from build123d import *

# Parameters (mm, degrees)
IZIM1_R                     = 125
Y_KSEKLIK_EKSTR_ZYON2_DEPTH = 400
IZIM2_R                     = 530
KES_EKSTR_ZYON1_DEPTH       = 150
IZIM3_R                     = 540
Y_KSEKLIK_EKSTR_ZYON3_DEPTH = 300


with BuildPart() as part:
    # Çizim1 → Yükseklik-Ekstrüzyon2 (new body)
    with BuildSketch(Plane(origin=(0, 0, 0), x_dir=(1, 0, 0), z_dir=(0, 1, 0))):
        with BuildLine():
            Line((-900, 700), (-900, -700))
            ThreePointArc((-900, -700), (-841.421356237, -841.421356237), (-700, -900))
            Line((-700, -900), (700, -900))
            ThreePointArc((700, -900), (841.421356237, -841.421356237), (900, -700))
            Line((900, -700), (900, 700))
            ThreePointArc((900, 700), (841.421356237, 841.421356237), (700, 900))
            Line((700, 900), (-700, 900))
            ThreePointArc((-700, 900), (-841.421356237, 841.421356237), (-900, 700))
        make_face()
        with Locations((-550, 550)):
            Circle(IZIM1_R, mode=Mode.SUBTRACT)
        with Locations((550, 550)):
            Circle(IZIM1_R, mode=Mode.SUBTRACT)
        with Locations((-550, -550)):
            Circle(IZIM1_R, mode=Mode.SUBTRACT)
        with Locations((550, -550)):
            Circle(IZIM1_R, mode=Mode.SUBTRACT)
    extrude(amount=Y_KSEKLIK_EKSTR_ZYON2_DEPTH)

    # Çizim2 → Kes-Ekstrüzyon1 (cut)
    with BuildSketch(Plane.XZ):
        Circle(IZIM2_R)
    extrude(amount=-KES_EKSTR_ZYON1_DEPTH, mode=Mode.SUBTRACT)

    # Çizim3 → Yükseklik-Ekstrüzyon3 (add)
    with BuildSketch(Plane.XZ.offset(-150)):
        Circle(IZIM3_R)
    extrude(amount=Y_KSEKLIK_EKSTR_ZYON3_DEPTH)


solid = part.part
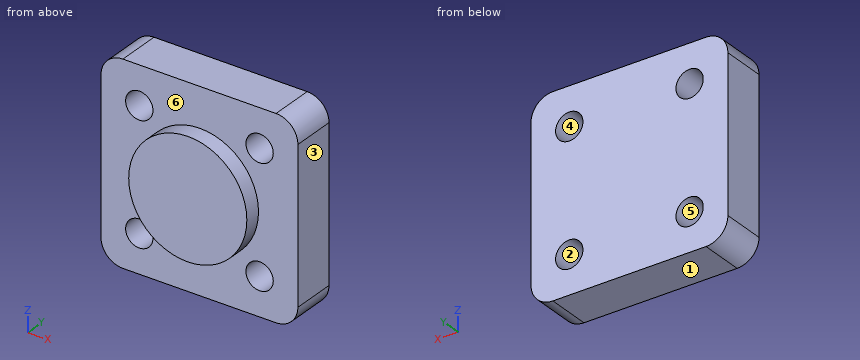
CAD build for the part. Positions are in the model's coordinates, mm. Face numbers are marked on the shaded views. A direction names the side the tool comes from. Coordinates: 2 decimals unless noted, no trailing zeros. Write each loop counter-clockwise with the first axis right and the second up, starting at its lowest first coordinate (ties: lowest second). Pieces come first, ordered by that corner, then holes. Notation, with made-up numbers: M 36.5,-29 L 45.5,-29 A7 ccw 45.5,-21 Z; hole C 71,50 d9. An arc over 180 degrees is marked long. Return JSON: item names as keys, results as strings.
Item 1: Slice it at C-C, the plane z = 288. Write the cut outline in (x, y).
Findings below:
{"outline": "M -900,0 L -456.79,0 L -456.79,-150 L 456.79,-150 L 456.79,0 L 900,0 L 900,400 L -900,400 Z"}
Item 2: Drop flat-ended pins along their axis: pin 1 Ø2 at (y, z) = (-77, -168) entering from -X; pin 2 Ø5 at (x, z) = (-351.5, -675) entering from -Y. Give the stop position or say it passes through.
Findings below:
{"pin 1": "stops at x = -513.53", "pin 2": "stops at y = 0"}
Item 3: Two-plate mould, pull along Z, no slides. Class the marked faces 1, 2, 3 and 4: +Z half, -Z half, draft (parallel to the pull), parting line (faces both ways), or undercut.
Findings below:
{"face 1": "-Z half", "face 2": "undercut", "face 3": "draft", "face 4": "undercut"}
Item 4: Probe line 1 (X direction, y = 132.5, z = -550.5); line 2 (X direction, y = 180, z = 503). List the from-to ranges inside material, lowest first. Write a range as from..to.
Findings below:
{"line 1": "x = -900..-675, -425..425, 675..900", "line 2": "x = -900..-665.83, -434.17..434.17, 665.83..900"}
Item 5: Which spindle directions (+Z, -Z, +X, -X, +Y, -Y) get a long thin tool onto all of the face, cutting with end or side? Do the marked faces 5 and 6. Say none if no direction does.
Findings below:
{"face 5": "+Y, -Y", "face 6": "-Y"}
Item 6: Slice it at A-A, the plane y = 49.5. Write the cut outline in (x, z).
Findings below:
{"outline": "M -900,-700 A200 ccw -700,-900 L 700,-900 A200 ccw 900,-700 L 900,700 A200 ccw 700,900 L -700,900 A200 ccw -900,700 Z; hole C -550,-550 d250; hole C -550,550 d250; hole C 550,-550 d250; hole C 550,550 d250"}
Item 7: Slice it at D-D, the plane y = -47. Write the cut outline in (x, z), and give its area (3 significant figures).
Findings below:
{"outline": "C 0,0 d1080", "area": "916,000 mm2"}
Item 8: Slice it at B-B, the plane x = 0. Write the cut outline in (y, z).
Findings below:
{"outline": "M -150,-540 L 0,-540 L 0,-900 L 400,-900 L 400,900 L 0,900 L 0,540 L -150,540 Z"}
